```python
from build123d import *

# Parameters (mm, degrees)
SKETCH1_R       = 4
EXTRUDE1_DEPTH  = 13
FILLET5_R       = 5
FILLET6_R       = 5
SKETCH8_R       = 4
EXTRUDE7_DEPTH  = 30
SKETCH9_W       = 42
SKETCH9_H       = 8
EXTRUDE8_DEPTH  = 42
EXTRUDE9_REACH  = 82
SKETCH10_R      = 11
SKETCH10_R_2    = 1.5
EXTRUDE10_REACH = 10
SKETCH11_W      = 21
SKETCH11_H      = 22
FILLET7_R       = 2.5


with BuildPart() as part:
    # Sketch1 → Extrude1 (new body)
    with BuildSketch(Plane(origin=(0, 0, 0), x_dir=(1, 0, 0), z_dir=(0, 1, 0))):
        Polygon((-26.25, -50), (30.331151632, -50), (30.331151632, -2.573593129), (-2.242441497, 30), (-21.668848368, 30), (-21.668848368, 0), (-14.668848368, 0), (0.331151632, -15), (0.331151632, -42), (-26.25, -42), align=None)
        with Locations((-8.786796564, 15)):
            Circle(SKETCH1_R, mode=Mode.SUBTRACT)
        with Locations((15, -8.786796564)):
            Circle(SKETCH1_R, mode=Mode.SUBTRACT)
    extrude(amount=EXTRUDE1_DEPTH)

    # Fillet5
    fillet5_edges = [part.edges().sort_by_distance(p)[0] for p in [
        (-2.242441497, 6.5, -30),
        (30.331151632, 6.5, 2.573593129),
        (30.331151632, 6.5, 50),
        (0.331151632, 6.5, 15),
        (-14.668848368, 6.5, 0),
    ]]
    fillet(fillet5_edges, radius=FILLET5_R)

    # Fillet6
    fillet6_edges = [part.edges().sort_by_distance(p)[0] for p in [
        (-21.668848368, 6.5, 0),
        (-21.668848368, 6.5, -30),
    ]]
    fillet(fillet6_edges, radius=FILLET6_R)

    # Sketch8 → Extrude7 (cut)
    with BuildSketch(Plane.ZY.offset(-0.331151632)):
        with Locations((28, 6.5)):
            Circle(SKETCH8_R)
    extrude(amount=-EXTRUDE7_DEPTH, mode=Mode.SUBTRACT)

    # Sketch9 → Extrude8 (add)
    with BuildSketch(Plane(origin=(0, 13, 0), x_dir=(-1, 0, 0), z_dir=(0, 1, 0))):
        with Locations((5.25, 46)):
            Rectangle(SKETCH9_W, SKETCH9_H)
    extrude(amount=EXTRUDE8_DEPTH)

    # Sketch10 → Extrude9 (cut, up to next)
    with BuildSketch(Plane.XY.offset(50), mode=Mode.PRIVATE) as extrude9_sk1:
        with Locations((-5.25, 34)):
            Circle(SKETCH10_R)
    extrude9_tool1 = extrude(extrude9_sk1.sketch, amount=-EXTRUDE9_REACH, mode=Mode.PRIVATE) & part.part
    add(extrude9_tool1.solids().sort_by_distance((-5.25, 34, 50))[0], mode=Mode.SUBTRACT)
    # Sketch10 → Extrude9 (cut, up to next)
    with BuildSketch(Plane.XY.offset(50), mode=Mode.PRIVATE) as extrude9_sk2:
        with Locations((10.25, 49.5)):
            Circle(SKETCH10_R_2)
    extrude9_tool2 = extrude(extrude9_sk2.sketch, amount=-EXTRUDE9_REACH, mode=Mode.PRIVATE) & part.part
    add(extrude9_tool2.solids().sort_by_distance((10.25, 49.5, 50))[0], mode=Mode.SUBTRACT)
    # Sketch10 → Extrude9 (cut, up to next)
    with BuildSketch(Plane.XY.offset(50), mode=Mode.PRIVATE) as extrude9_sk3:
        with Locations((-20.75, 49.5)):
            Circle(SKETCH10_R_2)
    extrude9_tool3 = extrude(extrude9_sk3.sketch, amount=-EXTRUDE9_REACH, mode=Mode.PRIVATE) & part.part
    add(extrude9_tool3.solids().sort_by_distance((-20.75, 49.5, 50))[0], mode=Mode.SUBTRACT)
    # Sketch10 → Extrude9 (cut, up to next)
    with BuildSketch(Plane.XY.offset(50), mode=Mode.PRIVATE) as extrude9_sk4:
        with Locations((-20.75, 18.5)):
            Circle(SKETCH10_R_2)
    extrude9_tool4 = extrude(extrude9_sk4.sketch, amount=-EXTRUDE9_REACH, mode=Mode.PRIVATE) & part.part
    add(extrude9_tool4.solids().sort_by_distance((-20.75, 18.5, 50))[0], mode=Mode.SUBTRACT)
    # Sketch10 → Extrude9 (cut, up to next)
    with BuildSketch(Plane.XY.offset(50), mode=Mode.PRIVATE) as extrude9_sk5:
        with Locations((10.25, 18.5)):
            Circle(SKETCH10_R_2)
    extrude9_tool5 = extrude(extrude9_sk5.sketch, amount=-EXTRUDE9_REACH, mode=Mode.PRIVATE) & part.part
    add(extrude9_tool5.solids().sort_by_distance((10.25, 18.5, 50))[0], mode=Mode.SUBTRACT)

    # Sketch11 → Extrude10 (cut, up to next)
    with BuildSketch(Plane(origin=(0, 0, 42), x_dir=(-1, 0, 0), z_dir=(0, 0, -1)), mode=Mode.PRIVATE) as extrude10_sk1:
        with Locations((-5.25, 34)):
            Rectangle(SKETCH11_W, SKETCH11_H)
    extrude10_tool1 = extrude(extrude10_sk1.sketch, amount=-EXTRUDE10_REACH, mode=Mode.PRIVATE) & part.part
    add(extrude10_tool1.solids().sort_by_distance((5.25, 34, 42))[0], mode=Mode.SUBTRACT)

    # Fillet7
    fillet7_edges = [part.edges().sort_by_distance(p)[0] for p in [
        (15.75, 23, 46),
        (15.75, 45, 46),
    ]]
    fillet(fillet7_edges, radius=FILLET7_R)


solid = part.part
```
Geometry check sheet. Reference: the model listing, model coordinates, mm. A direction names the side the tool comes from. Give positions to 0.01 mm unless a question says otherwise; leave off trailing zeros. Order: outer loops, then holes, each group sorted by start corner. A loop starts at its lowest first (then second) coordinate and runs counter-clockwise, first axis right, second up. Notation, with made-up numbers: (56, 15) - (114, 15) arc R24 ccw to (114, 40) - close; hole circle Ø10 at (44.5, 51.25). An arc over 180 degrees is marked (long way). Answer in a Markdown table with one row per item. Add a question column.
Q1. Mould release check, pull along Y, two halves, no side actions. Record for faces 5 (the cylindrical face through (-2.375, 6.591, -29.609)), 6 (the flat face through (10, 13, 9)), 7 (the cylindrical face through (9.925, 48.036, 46.056)): pulls with the +Y half, pulls with the -Y half, needs draft (parallel to the pull), parting line crosses it, or undercut.
Q2. Cross-section at A-A, the plane y = 49.5. Enter the section's corners in (x, z), then the cut area to 3 significant figures.
Q3. Cross-section at C-C, the plane z = -15. Enter the section's corners in (x, y), then the cut area to 3 significant figures.
Q4. Tool access check on faces 1 (the flat face through (-14, 27, 42)), 2 (the flat face through (15.75, 51, 46)), 3 (the cylindrical face through (15.037, 22.248, 46.056)), 4 (the cylindrical face through (-14.78, 6.59, 0.4)). Record the directions out of +Z, -Z, +X, -X, +Y, -Y that give a thin tool (end or side, any length) a straight path to the whole face; none if there is none.
Q5. Gauge pin test, flat ends, axial feed: pin 1 (2.5 mm diameter, centred on x = 10.25, y = 49.5, fed in from -Z); pin 2 (10.5 mm diameter, centred on x = 15, z = 8.79, fed in from -Y); pin 3 (4 mm diameter, centred on x = -20.75, y = 18.5, fed in from -Z); pin 4 (12 mm diameter, centred on y = 12, z = -14, fed in from +X). Record the tip position at first contact, or that the pin passes through.
Q6. Cross-section at B-B, the plane x = 2. Enter the section's corners in (y, z), then the cut area to 3 significant figures.
Q7. Material ranges on probe 1 along Y at (x, z) = (10, 45); probe 2 along Y at (x, z) = (15, 28); probe 3 along Z at (x, y) = (-17, 50.5), recorded low to high. Write a range as from..to.
Q8. Cross-section at D-D, the plane x = -10.5. Enter the section's corners in (y, z), then the cut area to 3 significant figures.
Check values:
| question | item | result |
|---|---|---|
| 1 | face 5 | needs draft |
| 1 | face 6 | pulls with the +Y half |
| 1 | face 7 | undercut |
| 2 | outline | (-26.25, 42) - (-22.25, 42) - (-22.25, 50) - (-26.25, 50) - close; (-19.25, 42) - (8.75, 42) - (8.75, 50) - (-19.25, 50) - close; (11.75, 42) - (15.75, 42) - (15.75, 50) - (11.75, 50) - close |
| 2 | area | 288 mm^2 |
| 3 | outline | (-21.67, 0) - (-12.79, 0) - (-12.79, 13) - (-21.67, 13) - close; (-4.79, 0) - (12.76, 0) - (12.76, 13) - (-4.79, 13) - close |
| 3 | area | 344 mm^2 |
| 4 | face 1 | -X, +Y |
| 4 | face 2 | +Z, -Z, +X, +Y |
| 4 | face 3 | +Z, -Z, +X |
| 4 | face 4 | -X, +Y, -Y |
| 5 | pin 1 | passes through |
| 5 | pin 2 | stops at y = 0 |
| 5 | pin 3 | stops at z = 42 |
| 5 | pin 4 | stops at x = 19.76 |
| 6 | outline | (0, -25.76) - (13, -25.76) - (13, 42) - (23, 42) - (23, 50) - (0, 50) - close; (45, 42) - (55, 42) - (55, 50) - (45, 50) - close; hole circle Ø8 at (6.5, 28) |
| 6 | area | 1,090 mm^2 |
| 7 | probe 1 | y = 0..17.02, 19.98..23, 45..48.02, 50.98..55 |
| 7 | probe 2 | y = 0..2.5, 10.5..13 |
| 7 | probe 3 | z = 42..50 |
| 8 | outline | (0, -30) - (13, -30) - (13, -18.61) - (0, -18.61) - close; (0, -11.39) - (13, -11.39) - (13, 4.17) - (0, 4.17) - close; (0, 42) - (24.33, 42) - (24.33, 50) - (0, 50) - close; (43.67, 42) - (55, 42) - (55, 50) - (43.67, 50) - close |
| 8 | area | 636 mm^2 |
